Check sheet for the modelled part. Datum: model origin and axes. Units: mm. A direction names the side the tool comes from. Coordinates: 2 decimals unless noted, no trailing zeros. Order: outer loops, then holes, each group sorted by start corner. A loop starts at its lowest first (then second) coordinate and runs counter-clockwise, first axis right, second up.
1. Cross-section at B-B (x = 8.5). Enter the section's corners in (y, z), then the cut area to 3 significant figures.
2. Thickness scan on line 1 (Z direction, x = 6.5, y = 24); line 2 (Z direction, x = 38, y = 6); line 3 (X direction, y = 9, z = -65). Record the ranges inside material, lowest first.
3. Set-up check for faces 4 (the flat face through (60.637, 21, -1)), 5 (the flat face through (0, 23, -80.709)): record each of +Z, -Z, +X, -X, +Y, -Y from which the full face is reachable in a straight line by a thin tool's end or side.
4. Gauge pin test, flat end, axial feed: pin 1 Ø0.6 at (x, z) = (55, 40.5) entering from +Y. Record the tip position at first contact, or that the pin passes through.
5. Draft check along Z on faces 1 (the flat face through (47.1, 8.048, -65.3)), 2 (the flat face through (-1, 21, -85.306)), 3 (the flat face through (-60.369, 21, 1)). Enter one of: released by +Z, released by -Z, zero draft, split by the parting line, or undercut.
6. Cross-section at A-A (z = -37.5). Enter the section's corners in (x, y).
```python
from build123d import *

# Parameters (mm, degrees)
BOSS_EXTRUDE1_DEPTH     = 41.656
CUT_EXTRUDE1_DEPTH      = 38.608
SKETCH7_R               = 1.5
BOSS_EXTRUDE2_DEPTH     = 5
MIRROR2_COPY_1_DEPTH    = 38.608
MIRROR2_COPY_2_SKETCH_R = 1.5
MIRROR2_COPY_2_DEPTH    = 5
BOSS_EXTRUDE3_START     = -2.9464
SKETCH9_W               = 1.27
SKETCH9_H               = 1.27
BOSS_EXTRUDE3_DEPTH     = 35.6616
BOSS_EXTRUDE4_START     = -2.9464
SKETCH10_W              = 1.27
SKETCH10_H              = 1.27
BOSS_EXTRUDE4_DEPTH     = 35.6616


with BuildPart() as part:
    # Sketch3 → Boss-Extrude1 (new body)
    with BuildSketch(Plane(origin=(0, 0, 0), x_dir=(1, 0, 0), z_dir=(0, 1, 0))):
        with BuildLine():
            Line((58.096932885, -85.686632753), (-57.828667115, -85.686632753))
            ThreePointArc((-57.828667115, -85.686632753), (-59.624718339, -84.942683977), (-60.368667115, -83.146632753))
            Line((-60.368667115, -83.146632753), (-60.368667115, 82.766167247))
            ThreePointArc((-60.368667115, 82.766167247), (-59.624718339, 84.562218471), (-57.828667115, 85.306167247))
            Line((-57.828667115, 85.306167247), (58.096932885, 85.306167247))
            ThreePointArc((58.096932885, 85.306167247), (59.892984109, 84.562218471), (60.636932885, 82.766167247))
            Line((60.636932885, 82.766167247), (60.636932885, -83.146632753))
            ThreePointArc((60.636932885, -83.146632753), (59.892984109, -84.942683977), (58.096932885, -85.686632753))
        make_face()
    extrude(amount=BOSS_EXTRUDE1_DEPTH)

    # Sketch6 → Cut-Extrude1 (cut)
    with BuildSketch(Plane(origin=(0, 41.656, 0), x_dir=(1, 0, 0), z_dir=(0, 1, 0))):
        with BuildLine():
            Line((-55.771267115, -0.190232753), (-55.771267115, 67.373392964))
            ThreePointArc((-55.771267115, 67.373392964), (-54.171667622, 71.235167754), (-50.309892833, 72.834767247))
            Line((-50.309892833, 72.834767247), (-36.517896511, 72.834767247))
            ThreePointArc((-36.517896511, 72.834767247), (-33.539782988, 73.959370118), (-32.04836951, 76.771767247))
            ThreePointArc((-32.04836951, 76.771767247), (-30.556956031, 79.584164375), (-27.578842508, 80.708767247))
            Line((-27.578842508, 80.708767247), (0.134132885, 80.708767247))
            Line((0.134132885, 80.708767247), (0.134132885, -0.190232753))
            Line((0.134132885, -0.190232753), (-55.771267115, -0.190232753))
        make_face()
    cut_extrude1 = extrude(amount=-CUT_EXTRUDE1_DEPTH, mode=Mode.SUBTRACT)

    # Sketch7 → Boss-Extrude2 (add)
    with BuildSketch(Plane(origin=(0, 3.048, 0), x_dir=(1, 0, 0), z_dir=(0, 1, 0))):
        with BuildLine():
            Line((-47.317674081, 67.712862285), (-47.317674081, 69.529651141))
            Line((-47.317674081, 69.529651141), (-44.630325919, 69.529651141))
            Line((-44.630325919, 69.529651141), (-44.630325919, 67.712862285))
            ThreePointArc((-44.630325919, 67.712862285), (-43.145219322, 66.773547925), (-42.205904962, 65.288441328))
            Line((-42.205904962, 65.288441328), (-40.389116105, 65.288441328))
            Line((-40.389116105, 65.288441328), (-40.389116105, 62.601093165))
            Line((-40.389116105, 62.601093165), (-42.205904962, 62.601093165))
            ThreePointArc((-42.205904962, 62.601093165), (-43.145219322, 61.115986569), (-44.630325919, 60.176672209))
            Line((-44.630325919, 60.176672209), (-44.630325919, 58.359883352))
            Line((-44.630325919, 58.359883352), (-47.317674081, 58.359883352))
            Line((-47.317674081, 58.359883352), (-47.317674081, 60.176672209))
            ThreePointArc((-47.317674081, 60.176672209), (-48.802780678, 61.115986569), (-49.742095038, 62.601093165))
            Line((-49.742095038, 62.601093165), (-51.558883895, 62.601093165))
            Line((-51.558883895, 62.601093165), (-51.558883895, 65.288441328))
            Line((-51.558883895, 65.288441328), (-49.742095038, 65.288441328))
            ThreePointArc((-49.742095038, 65.288441328), (-48.802780678, 66.773547925), (-47.317674081, 67.712862285))
        make_face()
        with Locations(Location((-45.974, 63.944767247, 0), (0, 0, 270))):
            Circle(SKETCH7_R, mode=Mode.SUBTRACT)
    boss_extrude2 = extrude(amount=BOSS_EXTRUDE2_DEPTH)

    # Mirror1: Cut-Extrude1, Boss-Extrude2 across plane
    add(cut_extrude1.mirror(Plane(origin=(0, 0, 0), x_dir=(0, 0, 1), z_dir=(1, 0, 0))), mode=Mode.SUBTRACT)
    add(boss_extrude2.mirror(Plane(origin=(0, 0, 0), x_dir=(0, 0, 1), z_dir=(1, 0, 0))))

    # Mirror2: Cut-Extrude1, Boss-Extrude2 across plane
    add(cut_extrude1.mirror(Plane.XY), mode=Mode.SUBTRACT)
    add(boss_extrude2.mirror(Plane.XY))

    # Mirror2 copy 1 sketch → Mirror2 copy 1 (cut)
    with BuildSketch(Plane(origin=(0, 41.656, 0), x_dir=(-1, 0, 0), z_dir=(0, 1, 0))):
        with BuildLine():
            Line((-55.771267115, -0.190232753), (-55.771267115, 67.373392964))
            ThreePointArc((-55.771267115, 67.373392964), (-54.171667622, 71.235167754), (-50.309892833, 72.834767247))
            Line((-50.309892833, 72.834767247), (-36.517896511, 72.834767247))
            ThreePointArc((-36.517896511, 72.834767247), (-33.539782988, 73.959370118), (-32.04836951, 76.771767247))
            ThreePointArc((-32.04836951, 76.771767247), (-30.556956031, 79.584164375), (-27.578842508, 80.708767247))
            Line((-27.578842508, 80.708767247), (0.134132885, 80.708767247))
            Line((0.134132885, 80.708767247), (0.134132885, -0.190232753))
            Line((0.134132885, -0.190232753), (-55.771267115, -0.190232753))
        make_face()
    extrude(amount=-MIRROR2_COPY_1_DEPTH, mode=Mode.SUBTRACT)

    # Mirror2 copy 2 sketch → Mirror2 copy 2 (add)
    with BuildSketch(Plane(origin=(0, 3.048, 0), x_dir=(-1, 0, 0), z_dir=(0, 1, 0))):
        with BuildLine():
            Line((-47.317674081, 67.712862285), (-47.317674081, 69.529651141))
            Line((-47.317674081, 69.529651141), (-44.630325919, 69.529651141))
            Line((-44.630325919, 69.529651141), (-44.630325919, 67.712862285))
            ThreePointArc((-44.630325919, 67.712862285), (-43.145219322, 66.773547925), (-42.205904962, 65.288441328))
            Line((-42.205904962, 65.288441328), (-40.389116105, 65.288441328))
            Line((-40.389116105, 65.288441328), (-40.389116105, 62.601093165))
            Line((-40.389116105, 62.601093165), (-42.205904962, 62.601093165))
            ThreePointArc((-42.205904962, 62.601093165), (-43.145219322, 61.115986569), (-44.630325919, 60.176672209))
            Line((-44.630325919, 60.176672209), (-44.630325919, 58.359883352))
            Line((-44.630325919, 58.359883352), (-47.317674081, 58.359883352))
            Line((-47.317674081, 58.359883352), (-47.317674081, 60.176672209))
            ThreePointArc((-47.317674081, 60.176672209), (-48.802780678, 61.115986569), (-49.742095038, 62.601093165))
            Line((-49.742095038, 62.601093165), (-51.558883895, 62.601093165))
            Line((-51.558883895, 62.601093165), (-51.558883895, 65.288441328))
            Line((-51.558883895, 65.288441328), (-49.742095038, 65.288441328))
            ThreePointArc((-49.742095038, 65.288441328), (-48.802780678, 66.773547925), (-47.317674081, 67.712862285))
        make_face()
        with Locations(Location((-45.974, 63.944767247, 0), (0, 0, 270))):
            Circle(MIRROR2_COPY_2_SKETCH_R, mode=Mode.SUBTRACT)
    extrude(amount=MIRROR2_COPY_2_DEPTH)

    # Sketch9 → Boss-Extrude3 (add)
    with BuildSketch(Plane(origin=(0, 41.656, 0), x_dir=(1, 0, 0), z_dir=(0, 1, 0)).offset(BOSS_EXTRUDE3_START)):
        with Locations((-1.7526, 80.073767247)):
            Rectangle(SKETCH9_W, SKETCH9_H)
        with Locations((1.7526, 80.073767247)):
            Rectangle(SKETCH9_W, SKETCH9_H)
    boss_extrude3 = extrude(amount=-BOSS_EXTRUDE3_DEPTH)

    # Mirror3: Boss-Extrude3 across plane
    add(boss_extrude3.mirror(Plane.XY))

    # Sketch10 → Boss-Extrude4 (add)
    with BuildSketch(Plane(origin=(0, 41.656, 0), x_dir=(1, 0, 0), z_dir=(0, 1, 0)).offset(BOSS_EXTRUDE4_START)):
        with Locations((55.136267115, -1.7526)):
            Rectangle(SKETCH10_W, SKETCH10_H)
        with Locations((55.136267115, 1.7526)):
            Rectangle(SKETCH10_W, SKETCH10_H)
        with Locations((55.136267115, 40.6654)):
            Rectangle(SKETCH10_W, SKETCH10_H)
        with Locations((55.136267115, 44.1706)):
            Rectangle(SKETCH10_W, SKETCH10_H)
        with Locations((55.136267115, -44.1706)):
            Rectangle(SKETCH10_W, SKETCH10_H)
        with Locations((55.136267115, -40.6654)):
            Rectangle(SKETCH10_W, SKETCH10_H)
    boss_extrude4 = extrude(amount=-BOSS_EXTRUDE4_DEPTH)

    # Mirror4: Boss-Extrude4 across plane
    add(boss_extrude4.mirror(Plane(origin=(0, 0, 0), x_dir=(0, 0, 1), z_dir=(1, 0, 0))))


solid = part.part
```
Data:
1. outline: (0, -85.31) - (41.66, -85.31) - (41.66, -80.71) - (3.05, -80.71) - (3.05, 80.71) - (41.66, 80.71) - (41.66, 85.69) - (0, 85.69) - close
1. area: 891 mm2
2. line 1: z = -85.31 to -80.71, 80.71 to 85.69
2. line 2: z = -85.31 to -72.83, 72.83 to 85.69
2. line 3: x = -60.37 to -55.77, 55.77 to 60.64
3. face 4: +Z, -Z, +X, +Y, -Y
3. face 5: +Y
4. pin 1: stops at y = 38.71
5. face 1: undercut
5. face 2: released by -Z
5. face 3: zero draft
6. outline: (-60.37, 0) - (60.64, 0) - (60.64, 41.66) - (55.77, 41.66) - (55.77, 3.05) - (-55.77, 3.05) - (-55.77, 41.66) - (-60.37, 41.66) - close
